Check sheet for the modelled part. Datum: model origin and axes. Units: mm. Face numbers are marked on the shaded views. A direction names the side the tool comes from. Round coordinates to 2 decimals unless told otherwise and drop trailing zeros. Order: outer loops, then holes, each group sorted by start corner. A loop starts at its lowest first (then second) coordinate and runs counter-clockwise, first axis right, second up. Notation, with made-up numbers: (33, -11.5) -> (42, -11.5) arc R19 cw to (42, 1.5) -> close; hole circle Ø5 at (2, 32.25). An arc over 180 degrees is marked (long way). Answer in a Markdown table with one row per item. Add a question column.
1. Sectioned sample at B-B, the plane x = -4.5. Record the boundary of the cut face in (y, z), then the cut area to 3 significant figures.
2. Access from +Z, -Z, +X, -X, +Y, -Y to the whole of each face (thin tool, end or side, straight path). Record for the marked faces 4, 5 and 6.
3. Depth check by flat-ended pin: P1, Ø2.5, axis at y = 21.5, z = 14, coming from the -X side; P2, Ø2, axis at x = -15, z = 15.5, coming from the -Y side; P3, Ø8, axis at x = 31, z = 11, coming from the -Y side; P4, Ø12, axis at y = -22, z = 18.5, coming from the +X side. Enter the tip coordinate at first touch or a pass-through.
4. Draft check along Y on the marked faces 1, 2 and 3. Enter one of: +Y half, -Y half, draft (parallel to the pull), parting line (faces both ways), or undercut.
5. Sectioned sample at D-D, the plane x = -35.5. Record the boundary of the cut face in (y, z), then the cut area to 3 significant figures.
6. Material ranges on L1, parallel to X at y = 18.5, z = -8.5; L2, parallel to Y at x = 5, z = 8; L3, parallel to X at y = 9, z = 6, recorded low to high. Write a range as from..to.
7. Sectioned sample at C-C, the plane y = 30. Record the boundary of the cut face in (x, z).
```python
from build123d import *

# Parameters (mm, degrees)
F1_DEPTH      = 2
F2_DEPTH      = 25
F3_W          = 5
F3_H          = 60
F4_DEPTH      = 15
F3_H_2        = 40
F5_DEPTH      = 15
F5_DEPTH_BACK = 1.5
F6_R          = 7
F8_DEPTH      = 86.001
F7_W          = 6.048347801
F7_H          = 1.5
F9_DEPTH      = 5.1
F10_W         = 6
F10_H         = 1.5
F11_DEPTH     = 5.1
F12_T1_DEPTH  = 41
F12_T3_DEPTH  = 40.980202511
F12_T8_DEPTH  = 53.480202511
F13_R         = 2


# Not quite as in the source:
# - a fillet or chamfer that OpenCascade refuses, or shapes differently, is made with other operations: its cross-section is extruded or revolved along the edge and cut away or added


with BuildPart() as f1:
    # F0 (on Top) → F1 (new body)
    with BuildSketch(Plane.XY):
        with BuildLine():
            ThreePointArc((40, 15.5), (39.4142135624, 16.9142135624), (38, 17.5))
            Line((38, 17.5), (15.75, 17.5))
            ThreePointArc((15.75, 17.5), (14.3357864376, 18.0857864376), (13.75, 19.5))
            Line((13.75, 19.5), (13.75, 22.5))
            ThreePointArc((13.75, 22.5), (13.4571067812, 23.2071067812), (12.75, 23.5))
            Line((12.75, 23.5), (-12.75, 23.5))
            ThreePointArc((-12.75, 23.5), (-13.4571067812, 23.2071067812), (-13.75, 22.5))
            Line((-13.75, 22.5), (-13.75, 19.5))
            ThreePointArc((-13.75, 19.5), (-14.3357864376, 18.0857864376), (-15.75, 17.5))
            Line((-15.75, 17.5), (-38, 17.5))
            ThreePointArc((-38, 17.5), (-39.4142135624, 16.9142135624), (-40, 15.5))
            Line((-40, 15.5), (-40, -15.5))
            ThreePointArc((-40, -15.5), (-39.4142135624, -16.9142135624), (-38, -17.5))
            Line((-38, -17.5), (-12, -17.5))
            ThreePointArc((-12, -17.5), (-11.4705903261, -17.5713410366), (-10.978949287, -17.7802746029))
            ThreePointArc((-10.978949287, -17.7802746029), (-10.4680840625, -16.8849116385), (-9.5, -16.5306922667))
            Line((-9.5, -16.5306922667), (0, -16.5306922667))
            Line((0, -16.5306922667), (9.5, -16.5306922667))
            ThreePointArc((9.5, -16.5306922667), (10.4680840625, -16.8849116385), (10.978949287, -17.7802746029))
            ThreePointArc((10.978949287, -17.7802746029), (11.4705903261, -17.5713410366), (12, -17.5))
            Line((12, -17.5), (38, -17.5))
            ThreePointArc((38, -17.5), (39.4142135624, -16.9142135624), (40, -15.5))
            Line((40, -15.5), (40, 15.5))
        make_face()
        with BuildLine():
            ThreePointArc((-9.5, 18.1578074247), (-11, 19.6578074247), (-9.5, 21.1578074247))
            Line((-9.5, 21.1578074247), (0, 21.1578074247))
            Line((0, 21.1578074247), (9.5, 21.1578074247))
            ThreePointArc((9.5, 21.1578074247), (11, 19.6578074247), (9.5, 18.1578074247))
            Line((9.5, 18.1578074247), (0, 18.1578074247))
            Line((0, 18.1578074247), (-9.5, 18.1578074247))
        make_face(mode=Mode.SUBTRACT)
    extrude(amount=F1_DEPTH)

    # F0 (on Top) → F2 (join)
    with BuildSketch(Plane.XY):
        with BuildLine():
            ThreePointArc((43, 18.5), (42.4142135624, 19.9142135624), (41, 20.5))
            Line((41, 20.5), (18.75, 20.5))
            ThreePointArc((18.75, 20.5), (17.3357864376, 21.0857864376), (16.75, 22.5))
            Line((16.75, 22.5), (16.75, 24.5))
            ThreePointArc((16.75, 24.5), (16.1642135624, 25.9142135624), (14.75, 26.5))
            Line((14.75, 26.5), (-14.75, 26.5))
            ThreePointArc((-14.75, 26.5), (-16.1642135624, 25.9142135624), (-16.75, 24.5))
            Line((-16.75, 24.5), (-16.75, 22.5))
            ThreePointArc((-16.75, 22.5), (-17.3357864376, 21.0857864376), (-18.75, 20.5))
            Line((-18.75, 20.5), (-41, 20.5))
            ThreePointArc((-41, 20.5), (-42.4142135624, 19.9142135624), (-43, 18.5))
            Line((-43, 18.5), (-43, -18.5))
            ThreePointArc((-43, -18.5), (-42.4142135624, -19.9142135624), (-41, -20.5))
            Line((-41, -20.5), (-15, -20.5))
            ThreePointArc((-15, -20.5), (-14, -20.7679491924), (-13.2679491924, -21.5))
            ThreePointArc((-13.2679491924, -21.5), (-12.5358983849, -22.2320508076), (-11.5358983849, -22.5))
            Line((-11.5358983849, -22.5), (11.5358983849, -22.5))
            ThreePointArc((11.5358983849, -22.5), (12.5358983849, -22.2320508076), (13.2679491924, -21.5))
            ThreePointArc((13.2679491924, -21.5), (14, -20.7679491924), (15, -20.5))
            Line((15, -20.5), (41, -20.5))
            ThreePointArc((41, -20.5), (42.4142135624, -19.9142135624), (43, -18.5))
            Line((43, -18.5), (43, 18.5))
        make_face()
        with BuildLine():
            Line((15.75, 17.5), (38, 17.5))
            ThreePointArc((38, 17.5), (39.4142135624, 16.9142135624), (40, 15.5))
            Line((40, 15.5), (40, -15.5))
            ThreePointArc((40, -15.5), (39.4142135624, -16.9142135624), (38, -17.5))
            Line((38, -17.5), (12, -17.5))
            ThreePointArc((12, -17.5), (11.4705903261, -17.5713410366), (10.978949287, -17.7802746029))
            ThreePointArc((10.978949287, -17.7802746029), (10.4542270396, -18.2309113684), (10.1143819168, -18.8333333333))
            ThreePointArc((10.1143819168, -18.8333333333), (9.7489231444, -19.3164965809), (9.1715728753, -19.5))
            Line((9.1715728753, -19.5), (0, -19.5))
            Line((0, -19.5), (-9.1715728753, -19.5))
            Line((-9.1715728753, -19.5), (-9.1981146163, -19.5))
            ThreePointArc((-9.1981146163, -19.5), (-9.1973546351, -19.4998436487), (-9.1965947349, -19.4996869043))
            ThreePointArc((-9.1965947349, -19.4996869043), (-9.7590938823, -19.3092089139), (-10.1143819168, -18.8333333333))
            ThreePointArc((-10.1143819168, -18.8333333333), (-10.4542270396, -18.2309113684), (-10.978949287, -17.7802746029))
            ThreePointArc((-10.978949287, -17.7802746029), (-11.4705903261, -17.5713410366), (-12, -17.5))
            Line((-12, -17.5), (-38, -17.5))
            ThreePointArc((-38, -17.5), (-39.4142135624, -16.9142135624), (-40, -15.5))
            Line((-40, -15.5), (-40, 15.5))
            ThreePointArc((-40, 15.5), (-39.4142135624, 16.9142135624), (-38, 17.5))
            Line((-38, 17.5), (-15.75, 17.5))
            ThreePointArc((-15.75, 17.5), (-14.3357864376, 18.0857864376), (-13.75, 19.5))
            Line((-13.75, 19.5), (-13.75, 22.5))
            ThreePointArc((-13.75, 22.5), (-13.4571067812, 23.2071067812), (-12.75, 23.5))
            Line((-12.75, 23.5), (12.75, 23.5))
            ThreePointArc((12.75, 23.5), (13.4571067812, 23.2071067812), (13.75, 22.5))
            Line((13.75, 22.5), (13.75, 19.5))
            ThreePointArc((13.75, 19.5), (14.3357864376, 18.0857864376), (15.75, 17.5))
        make_face(mode=Mode.SUBTRACT)
    extrude(amount=F2_DEPTH)

    # F3 (on Top) → F4 (join)
    with BuildSketch(Plane.XY):
        with Locations((-40.5, -30)):
            Rectangle(F3_W, F3_H)
        with Locations((40.5, -30)):
            Rectangle(F3_W, F3_H)
    extrude(amount=-F4_DEPTH)

    # F3 (on Top) → F5 (join, two sides)
    with BuildSketch(Plane.XY) as f5_sk:
        with Locations((-40.5, 20)):
            Rectangle(F3_W, F3_H_2)
        with Locations((40.5, 20)):
            Rectangle(F3_W, F3_H_2)
    extrude(amount=-F5_DEPTH)
    extrude(f5_sk.sketch, amount=F5_DEPTH_BACK)

    # F6
    f6_edges = [f1.edges().sort_by_distance(p)[0] for p in [
        (40.5, 40, -15),
        (-40.5, 40, -15),
        (-40.5, -60, -15),
        (40.5, -60, -15),
    ]]
    fillet(f6_edges, radius=F6_R)

    # F7 (on face) → F8 (cut, through all)
    with BuildSketch(Plane(origin=(-43, 0, 0), x_dir=(0, -1, 0), z_dir=(-1, 0, 0))):
        with BuildLine():
            Line((-26.5285503119, 1.5), (-40, 1.5))
            add(Edge.make_bspline(
                [(-40, 1.5), (-39.5081001265, 1.219408998), (-38.2821576057, 0.5201031862), (-35.7543121769, 0.1947861269), (-34.240745008, 0)],
                knots=[0, 0, 0, 0, 0.4012421995, 1, 1, 1, 1], degree=3))
            Line((-34.240745008, 0), (-26.5285503119, 0))
            Line((-26.5285503119, 0), (-26.5285503119, 1.5))
        make_face()
    extrude(amount=-F8_DEPTH, mode=Mode.SUBTRACT)

    # F7 (on face) → F9 (cut)
    with BuildSketch(Plane(origin=(-43, 0, 0), x_dir=(0, -1, 0), z_dir=(-1, 0, 0))):
        with Locations((-23.5043764114, 0.75)):
            Rectangle(F7_W, F7_H)
    extrude(amount=-F9_DEPTH, mode=Mode.SUBTRACT)

    # F10 (on face) → F11 (cut)
    with BuildSketch(Plane.YZ.offset(43)):
        with Locations((23.5285503119, 0.75)):
            Rectangle(F10_W, F10_H)
    extrude(amount=-F11_DEPTH, mode=Mode.SUBTRACT)

    # F12: fillet of radius 5 on 2 edges, made by hand

    # F12_s2 → F12_t1 (join)
    with BuildSketch(Plane.XZ.offset(-20.5)):
        with BuildLine():
            ThreePointArc((38, -5), (36.5355339059, -1.4644660941), (33, 0))
            Line((33, 0), (38, 0))
            Line((38, 0), (38, -5))
        make_face()
    extrude(amount=F12_T1_DEPTH)

    # F12_s4 → F12_t3 (join)
    with BuildSketch(Plane.XZ.offset(-20.480202511)):
        with BuildLine():
            ThreePointArc((-38, -5), (-36.5355339059, -1.4644660941), (-33, 0))
            Line((-33, 0), (-38, 0))
            Line((-38, 0), (-38, -5))
        make_face()
    extrude(amount=F12_T3_DEPTH)


with BuildPart() as f12_tool6:
    # F12_s7 → F12_t8 (new body)
    with BuildSketch(Plane.XZ.offset(20.5)):
        with BuildLine():
            ThreePointArc((-38, -5), (-36.5355339059, -1.4644660941), (-33, 0))
            Line((-33, 0), (-38, 0))
            Line((-38, 0), (-38, -5))
        make_face()
    extrude(amount=-F12_T8_DEPTH)

    split(bisect_by=Plane.XZ.offset(-20.5), keep=Keep.TOP)

    split(bisect_by=Plane.YZ.offset(-37.9), keep=Keep.TOP)


with BuildPart() as f1_1:
    add(f1.part)

    # F12_t5: union F12_tool6
    add(f12_tool6.part)

    # F13
    f13_edges = [f1_1.edges().sort_by_distance(p)[0] for p in [
        (-38, 40, -3.25),
        (-43, 40, -3.25),
        (38, 40, -3.25),
        (43, 40, -3.25),
        (43, 37.949747, -12.949747),
        (43, -10, -15),
        (43, -57.949747, -12.949747),
        (43, -60, -4),
        (38, -57.949747, -12.949747),
        (38, -60, -4),
        (38, 37.949747, -12.949747),
        (38, -10, -15),
        (-38, -60, -4),
        (-38, 37.949747, -12.949747),
        (-38, -10, -15),
        (-38, -57.949747, -12.949747),
        (-43, -57.949747, -12.949747),
        (-43, -10, -15),
        (-43, 37.949747, -12.949747),
        (-43, -60, -4),
    ]]
    fillet(f13_edges, radius=F13_R)


solid = f1_1.part
```
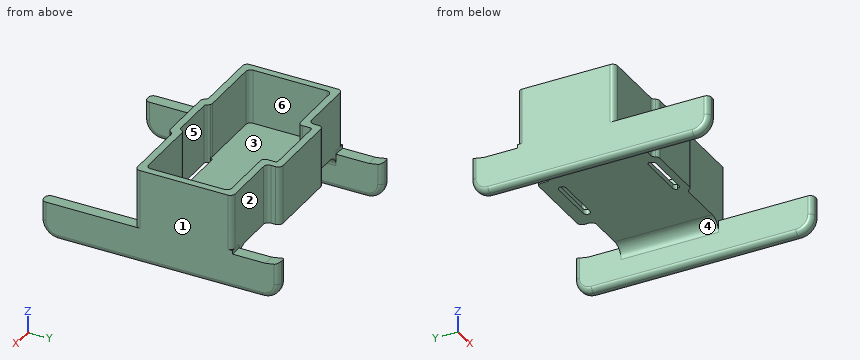
Answer key:
| question | item | result |
|---|---|---|
| 1 | outline | (-22.5, 0) -> (-19.5, 0) -> (-19.5, 25) -> (-22.5, 25) -> close; (-16.53, 0) -> (18.16, 0) -> (18.16, 2) -> (-16.53, 2) -> close; (21.16, 0) -> (26.5, 0) -> (26.5, 25) -> (23.5, 25) -> (23.5, 2) -> (21.16, 2) -> close |
| 1 | area | 224 mm² |
| 2 | face 4 | -Z, +Y, -Y |
| 2 | face 5 | +Z, -Z |
| 2 | face 6 | +Z |
| 3 | P1 | stops at x = -41.97 |
| 3 | P2 | stops at y = -20.77 |
| 3 | P3 | stops at y = -20.5 |
| 3 | P4 | stops at x = 43 |
| 4 | face 1 | draft |
| 4 | face 2 | +Y half |
| 4 | face 3 | undercut |
| 5 | outline | (-20.5, -0.67) -> (20.5, -0.67) -> (20.5, 25) -> (17.5, 25) -> (17.5, 2) -> (-17.5, 2) -> (-17.5, 25) -> (-20.5, 25) -> close |
| 5 | area | 247 mm² |
| 6 | L1 | x = -43..-38, 38..43 |
| 6 | L2 | y = -22.5..-19.5, 23.5..26.5 |
| 6 | L3 | x = -43..-40, 40..43 |
| 7 | outline | (-43, -13) arc R2 ccw to (-41, -15) -> (-40, -15) arc R2 ccw to (-38, -13) -> (-38, 0) -> (-43, 0) -> close; (38, -13) arc R2 ccw to (40, -15) -> (41, -15) arc R2 ccw to (43, -13) -> (43, 0) -> (38, 0) -> close |
